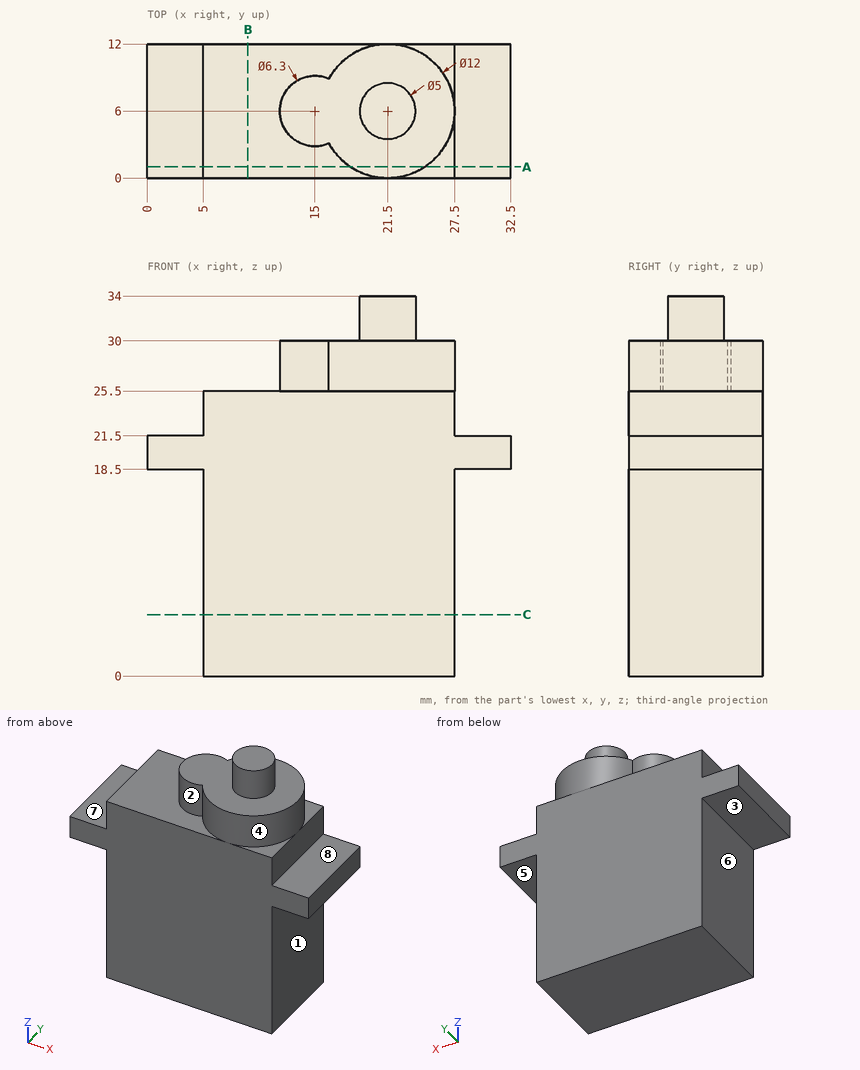
Check sheet for the drawn part. Datum: minimum x, y, z corner. Units: mm. A direction names the side the tool comes from. Round coordinates to 2 decimals unless told otherwise and drop trailing zeros. Loops run counter-clockwise (first coordinate to the right, second up) from the corner with the lowest first, then second, coordinate; pieces in that order, holes last. Notation, with made-up numbers: (74.25, 0.25) - (85.25, 0.25) arc R36 cw to (85.25, 39.25) - close; hole circle Ø6 at (83, 14.5). An arc over 180 degrees is marked (long way). Write item = value, one per line. Start each with the question number.
1. Set-up check for the marked faces 4, 5, 6, 7 and 8: record each of +Z, -Z, +X, -X, +Y, -Y from which the full face is reachable in a straight line by a thin tool's end or side.
2. Section check B-B on x = 9. Enter the section's corners in (y, z), then the cut area to 3 significant figures.
3. Depth check by flat-ended pin: pin 1 (1.8 mm diameter, centred on x = 25, y = 4, fed in from +Z); pin 2 (6 mm diameter, centred on y = 4, z = 10, fed in from +X); pin 3 (3.5 mm diameter, centred on y = 4.5, z = 10, fed in from -X). Enter the tip coordinate at first touch or a pass-through.
4. Section check A-A on y = 1. Enter the section's corners in (x, z), then the cut area to 3 significant figures.
5. Mould release check, pull along X, two halves, no side actions. Record for the marked faces 1, 2 and 3: released by +X, released by -X, zero draft, split by the parting line, or undercut.
6. Thickness scan on line 1 (Z direction, x = 15, y = 6.5); line 2 (X direction, y = 6.25, z = 17); line 3 (Z direction, x = 7.5, y = 6.5). Record the ranges inside material, lowest first.
7. Section check C-C on z = 5.5. Enter the section's corners in (x, y), then the cut area to 3 significant figures.
Working result:
q1.face_4 = +Z
q1.face_5 = -Z, +X, +Y, -Y
q1.face_6 = -Z, -X, +Y, -Y
q1.face_7 = +Z, -X, +Y, -Y
q1.face_8 = +Z, +X, +Y, -Y
q2.outline = (0, 0) - (12, 0) - (12, 25.5) - (0, 25.5) - close
q2.area = 306 mm^2
q3.pin_1 = 30
q3.pin_2 = 27.5
q3.pin_3 = 5
q4.outline = (0, 18.5) - (5, 18.5) - (5, 0) - (27.5, 0) - (27.5, 18.5) - (32.5, 18.5) - (32.5, 21.5) - (27.5, 21.5) - (27.5, 25.5) - (24.82, 25.5) - (24.82, 30) - (18.18, 30) - (18.18, 25.5) - (5, 25.5) - (5, 21.5) - (0, 21.5) - close
q4.area = 634 mm^2
q5.face_1 = released by +X
q5.face_2 = undercut
q5.face_3 = zero draft
q6.line_1 = 0 to 30
q6.line_2 = 5 to 27.5
q6.line_3 = 0 to 25.5
q7.outline = (5, 0) - (27.5, 0) - (27.5, 12) - (5, 12) - close
q7.area = 270 mm^2
